Work out the finished part from the listing and answer in its coordinate system (mm). A direction names the side the tool comes from. Coordinates: 2 decimals unless noted, no trailing zeros. Write each loop counter-clockwise with the first axis right and the second up, starting at its lowest first coordinate (ties: lowest second). Pieces come first, ordered by that corner, then holes. Notation, with made-up numbers: M 69.25,26.25 L 125.25,26.25 A21 cw 125.25,63.25 Z; hole C 14,-32.75 d11. An arc over 180 degrees is marked long. Use CSV: the item, a comma, the result in double quotes.
from build123d import *

# Parameters (mm, degrees)
SKETCH_1_R           = 41.2
EXTRUDE_1_DEPTH      = 20
EXTRUDE_3_DEPTH      = 15.2
EXTRUDE_3_DEPTH_BACK = 32.2
SKETCH_2_W           = 82.4
SKETCH_2_H           = 30
SKETCH_3_OUTSIDE_W   = 113.996
SKETCH_3_OUTSIDE_H   = 113.996
SKETCH_3_OUTSIDE_R   = 41.2
CUT_EXTRUDE_1_DEPTH  = 70.2
SKETCH_4_R           = 20
CUT_EXTRUDE_2_DEPTH  = 43.8
SKETCH_5_R           = 15.7
CUT_EXTRUDE_3_DEPTH  = 3.6
SKETCH_9_R           = 35.2
CUT_EXTRUDE_6_DEPTH  = 10
SKETCH_10_R          = 29.2
CUT_EXTRUDE_7_DEPTH  = 10
SKETCH_12_R          = 2
CUT_EXTRUDE_8_DEPTH  = 10
SKETCH_13_R          = 2
CUT_EXTRUDE_9_DEPTH  = 2.1
SKETCH_15_R          = 0.8
CUT_EXTRUDE_10_DEPTH = 1.5
SKETCH_16_R          = 2
CUT_EXTRUDE_13_DEPTH = 40


with BuildPart() as part:
    # 草图1 → 凸台-拉伸1 (new body)
    with BuildSketch(Plane.XY):
        Circle(SKETCH_1_R)
    extrude(amount=EXTRUDE_1_DEPTH)

    # 草图2 → 凸台-拉伸3 (add, two sides: drawn at the far end of the back side and taken through both)
    with BuildSketch(Plane(origin=(0, 0, 0), x_dir=(1, 0, 0), z_dir=(0, 1, 0)).offset(-EXTRUDE_3_DEPTH_BACK)):
        with Locations((0, 15)):
            Rectangle(SKETCH_2_W, SKETCH_2_H)
        with BuildLine():
            Line((-41.2, 30), (41.2, 30))
            ThreePointArc((41.2, 30), (0, 71.2), (-41.2, 30))
        make_face()
    extrude(amount=EXTRUDE_3_DEPTH + EXTRUDE_3_DEPTH_BACK)

    # 草图3 outside → 切除-拉伸1 (cut)
    with BuildSketch(Plane(origin=(0, 0, 0), x_dir=(-1, 0, 0), z_dir=(0, 0, -1))):
        Rectangle(SKETCH_3_OUTSIDE_W, SKETCH_3_OUTSIDE_H)
        with Locations(Location((0, 0, 0), (0, 0, 180))):
            Circle(SKETCH_3_OUTSIDE_R, mode=Mode.SUBTRACT)
    extrude(amount=CUT_EXTRUDE_1_DEPTH, mode=Mode.SUBTRACT)

    # 草图4 → 切除-拉伸2 (cut)
    with BuildSketch(Plane(origin=(0, 15.2, 0), x_dir=(1, 0, 0), z_dir=(0, 1, 0))):
        with Locations(Location((0, 30, 0), (0, 0, 270))):
            Circle(SKETCH_4_R)
    extrude(amount=-CUT_EXTRUDE_2_DEPTH, mode=Mode.SUBTRACT)

    # 草图5 → 切除-拉伸3 (cut)
    with BuildSketch(Plane(origin=(0, -28.6, 0), x_dir=(1, 0, 0), z_dir=(0, 1, 0))):
        with Locations(Location((0, 30, 0), (0, 0, 270))):
            Circle(SKETCH_5_R)
    extrude(amount=-CUT_EXTRUDE_3_DEPTH, mode=Mode.SUBTRACT)

    # 草图9 → 切除-拉伸6 (cut)
    with BuildSketch(Plane.XY.offset(20)):
        Circle(SKETCH_9_R)
    extrude(amount=-CUT_EXTRUDE_6_DEPTH, mode=Mode.SUBTRACT)

    # 草图10 → 切除-拉伸7 (cut)
    with BuildSketch(Plane.XY.offset(10)):
        Circle(SKETCH_10_R)
    extrude(amount=-CUT_EXTRUDE_7_DEPTH, mode=Mode.SUBTRACT)

    # 草图12 → 切除-拉伸8 (cut)
    with BuildSketch(Plane.XY):
        with Locations((-25, 20)):
            Circle(SKETCH_12_R)
        with Locations((-17, 28)):
            Circle(SKETCH_12_R)
        with Locations((25, 20)):
            Circle(SKETCH_12_R)
        with Locations((17, 28)):
            Circle(SKETCH_12_R)
    extrude(amount=CUT_EXTRUDE_8_DEPTH, mode=Mode.SUBTRACT)

    # 草图13 → 切除-拉伸9 (cut)
    with BuildSketch(Plane.XZ.offset(32.2)):
        with Locations(Location((0, -48, 0), (0, 0, 270))):
            Circle(SKETCH_13_R)
        with Locations(Location((-12.727922061, -42.727922061, 0), (0, 0, 270))):
            Circle(SKETCH_13_R)
        with Locations(Location((-18, -30, 0), (0, 0, 270))):
            Circle(SKETCH_13_R)
        with Locations(Location((-12.727922061, -17.272077939, 0), (0, 0, 270))):
            Circle(SKETCH_13_R)
        with Locations(Location((0, -12, 0), (0, 0, 270))):
            Circle(SKETCH_13_R)
        with Locations(Location((12.727922061, -17.272077939, 0), (0, 0, 270))):
            Circle(SKETCH_13_R)
        with Locations(Location((18, -30, 0), (0, 0, 270))):
            Circle(SKETCH_13_R)
        with Locations(Location((12.727922061, -42.727922061, 0), (0, 0, 270))):
            Circle(SKETCH_13_R)
    extrude(amount=-CUT_EXTRUDE_9_DEPTH, mode=Mode.SUBTRACT)

    # 草图15 → 切除-拉伸10 (cut)
    with BuildSketch(Plane(origin=(0, -30.1, 0), x_dir=(-1, 0, 0), z_dir=(0, -1, 0))):
        with Locations(Location((0, 48, 0), (0, 0, 90))):
            Circle(SKETCH_15_R)
        with Locations(Location((12.727922061, 42.727922061, 0), (0, 0, 90))):
            Circle(SKETCH_15_R)
        with Locations(Location((18, 30, 0), (0, 0, 90))):
            Circle(SKETCH_15_R)
        with Locations(Location((12.727922061, 17.272077939, 0), (0, 0, 90))):
            Circle(SKETCH_15_R)
        with Locations(Location((0, 12, 0), (0, 0, 90))):
            Circle(SKETCH_15_R)
        with Locations(Location((-12.727922061, 17.272077939, 0), (0, 0, 90))):
            Circle(SKETCH_15_R)
        with Locations(Location((-18, 30, 0), (0, 0, 90))):
            Circle(SKETCH_15_R)
        with Locations(Location((-12.727922061, 42.727922061, 0), (0, 0, 90))):
            Circle(SKETCH_15_R)
    extrude(amount=-CUT_EXTRUDE_10_DEPTH, mode=Mode.SUBTRACT)

    # 草图16 → 切除-拉伸13 (cut)
    with BuildSketch(Plane(origin=(0, 15.2, 0), x_dir=(1, 0, 0), z_dir=(0, 1, 0))):
        with Locations(Location((-17.5, 47.5, 0), (0, 0, 270))):
            Circle(SKETCH_16_R)
        with Locations(Location((17.5, 47.5, 0), (0, 0, 270))):
            Circle(SKETCH_16_R)
    extrude(amount=-CUT_EXTRUDE_13_DEPTH, mode=Mode.SUBTRACT)


solid = part.part
Item 1: The part is cut by section C-C (y = 28). Write down the section's boundary in (x, z).
Answer:
outline,"M -30.22,0 L -19,0 L -19,10 L -21.33,10 L -21.33,20 L -30.22,20 Z; M -15,0 L -8.28,0 L -8.28,10 L -15,10 Z; M 8.28,0 L 15,0 L 15,10 L 8.28,10 Z; M 19,0 L 30.22,0 L 30.22,20 L 21.33,20 L 21.33,10 L 19,10 Z"
Item 2: A tool of negligible diameter and unlimited length cuts with its end or side. For faces 4 (the face through (0, -32.2, -52)), 5 (the face through (-1, -30.1, -48)), 6 (the face through (-21, -21, 10)), 7 (the face through (17, 26, 5)), 8 (the face through (18, -24.8, -48)), from which of +Z, -Z, +X, -X, +Y, -Y can it reach the whole face along a straight path? Write none if from no direction.
Answer:
face 4,"-Z, +X, -X, -Y"
face 5,"-Y"
face 6,"+Z"
face 7,"+Z, -Z"
face 8,"+Y"
Item 3: The part is cut by section B-B (x = -8). Write down the section's boundary in (y, z), then the cut area to 3 significant figures.
Answer:
outline,"M -40.42,0 L -32.2,0 L -32.2,-16.49 L -28.6,-16.49 L -28.6,-11.67 L 15.2,-11.67 L 15.2,0 L -28.08,0 L -28.08,10 L -34.28,10 L -34.28,20 L -40.42,20 Z; M -32.2,-70.42 L 15.2,-70.42 L 15.2,-48.33 L -28.6,-48.33 L -28.6,-43.51 L -32.2,-43.51 Z; M 28.08,0 L 40.42,0 L 40.42,20 L 34.28,20 L 34.28,10 L 28.08,10 Z"
area,"2,000 mm2"
Item 4: The part is cut by section D-D (z = 2.5). Write down the section's boundary in (x, y), then the cut area to 3 significant figures.
Answer:
outline,"C 0,0 d82.4; hole C 0,0 d58.4; hole C -25,20 d4; hole C -17,28 d4; hole C 17,28 d4; hole C 25,20 d4"
area,"2,600 mm2"
Item 5: Consider probe 1 along X at (y, z) = (-16.5, -48); probe 2 along X at (y, z) = (-9, -47); probe 3 along Y at (x, z) = (0, 4.5). Determine where each line is inside the solid, lowest interval first.
Answer:
probe 1,"x = -37.06 to -19.44, -15.56 to -8.72, 8.72 to 15.56, 19.44 to 37.06"
probe 2,"x = -37.53 to -19.44, -15.56 to -10.54, 10.54 to 15.56, 19.44 to 37.53"
probe 3,"y = -41.2 to -29.2, 29.2 to 41.2"
Item 6: Given pin 1 (8 mm diameter, centred on x = -20.5, y = 8, fed in from +Z); pin 2 (1.8 mm diameter, centred on x = -12.73, z = -42.73, fed in from +Y); pin 3 (3 mm diameter, centred on x = -12.73, z = -42.73, fed in from -Y), each flat-ended and moving along its own axis, determine where each tip first touches the part or whether it passes through.
Answer:
pin 1,"stops at z = 0"
pin 2,"stops at y = -28.6"
pin 3,"stops at y = -30.1"
Item 7: For a pull along Y with two mould halves and no side action, classify faces 1 (the face through (33.575, 10.573, 15.07)), 2 (the face through (30, 19, 20)), 3 (the face through (-17, -24.8, -48)) as released by +Y, released by -Y, zero draft, split by the parting line, or undercut.
Answer:
face 1,"undercut"
face 2,"zero draft"
face 3,"released by +Y"
Item 8: The part is cut by section A-A (z = -37.5). Write down the section's boundary in (x, y).
Answer:
outline,"M -40.51,-7.5 A41.2 ccw -25.7,-32.2 L -13.79,-32.2 L -13.79,-28.6 L -18.54,-28.6 L -18.54,15.2 L -38.29,15.2 A41.2 ccw -40.51,7.5 Z; M 13.79,-32.2 L 25.7,-32.2 A41.2 ccw 40.51,-7.5 L 40.51,7.5 A41.2 ccw 38.29,15.2 L 18.54,15.2 L 18.54,-28.6 L 13.79,-28.6 Z"
